from build123d import *

# Parameters (mm, degrees)
SKETCH1_W                                           = 160
SKETCH1_H                                           = 80
BOSS_EXTRUDE1_DEPTH                                 = 15
CBORE_FOR_M5_HEX_SOCKET_HEAD_CAP_SCREW1_D           = 5.5
CBORE_FOR_M5_HEX_SOCKET_HEAD_CAP_SCREW1_CBORE_D     = 10
CBORE_FOR_M5_HEX_SOCKET_HEAD_CAP_SCREW1_CBORE_DEPTH = 5.4
M6_TAPPED_HOLE1_D                                   = 5
SKETCH15_W                                          = 40
SKETCH15_H                                          = 80
SKETCH15_W_2                                        = 50
CUT_EXTRUDE1_DEPTH                                  = 2


with BuildPart() as part:
    # Sketch1 → Boss-Extrude1 (new body)
    with BuildSketch(Plane.XY):
        Rectangle(SKETCH1_W, SKETCH1_H)
    extrude(amount=BOSS_EXTRUDE1_DEPTH)

    # CBORE for M5 Hex Socket Head Cap Screw1 (through all)
    with Locations(Plane(origin=(74, 31, 0), x_dir=(-1, 0, 0), z_dir=(0, 0, -1))):
        with Locations((0, 0), (28, 0), (0, -21), (28, -21), (0, -41), (0, -62), (28, -41), (28, -62), (56, -41), (56, -21), (92, -21), (92, -41), (120, 0), (120, -21), (148, 0), (148, -21), (120, -41), (120, -62), (148, -41), (148, -62)):
            CounterBoreHole(CBORE_FOR_M5_HEX_SOCKET_HEAD_CAP_SCREW1_D / 2, CBORE_FOR_M5_HEX_SOCKET_HEAD_CAP_SCREW1_CBORE_D / 2, CBORE_FOR_M5_HEX_SOCKET_HEAD_CAP_SCREW1_CBORE_DEPTH)

    # M6 Tapped Hole1 (through all)
    with Locations(Plane(origin=(-60, -40, 7.5), x_dir=(0, 0, -1), z_dir=(0, -1, 0))):
        with Locations((0, 0), (0, 120)):
            Hole(M6_TAPPED_HOLE1_D / 2)

    # Sketch15 → Cut-Extrude1 (cut)
    with BuildSketch(Plane.XY.offset(15)):
        with Locations((-60, 0)):
            Rectangle(SKETCH15_W, SKETCH15_H)
        with Locations((60, 0)):
            Rectangle(SKETCH15_W, SKETCH15_H)
        Rectangle(SKETCH15_W_2, SKETCH15_H)
    extrude(amount=-CUT_EXTRUDE1_DEPTH, mode=Mode.SUBTRACT)


solid = part.part
The listing builds one solid part. Answer for the finished solid, in the listing's coordinates (mm). A direction names the side the tool comes from. Round coordinates to 2 decimals unless told otherwise and drop trailing zeros. Loops run counter-clockwise (first coordinate to the right, second up) from the corner with the lowest first, then second, coordinate; pieces in that order, holes last. Notation, with made-up numbers: M 74,37.5 L 113,37.5 A11 cw 113,52.5 Z; hole C 21,1.25 d5. An arc over 180 degrees is marked long. Return JSON: item names as keys, results as strings.
Q1. Find section A-A, the plane x = 60. Determine the outline of the cut face in (y, z), plus the area to 3 significant figures.
Results list:
{"outline": "M -40,0 L 40,0 L 40,5 L -40,5 Z; M -40,10 L 40,10 L 40,13 L -40,13 Z", "area": "640 mm2"}
Q2. Find the intervals of material crossed by line 1 along X through (y, z) = (31.5, 1.75); line 2 along Y through (x, z) = (-17.5, 2.25); line 3 along X through (y, z) = (1.5, 7.5), in increasing order. Write a range as from..to.
Results list:
{"line 1": "x = -80..-78.97, -69.03..-50.97, -41.03..41.03, 50.97..69.03, 78.97..80", "line 2": "y = -40..-14.97, -5.03..5.03, 14.97..40", "line 3": "x = -80..-62.5, -57.5..57.5, 62.5..80"}
Q3. The mould has two halves that part along Y. Classify faces 4 (the face through (-42, 13, 3)), 5 (the face through (-1, 40, 7)), 6 (the face through (32, 1, 15)): released by +Y, released by -Y, zero draft, split by the parting line, or undercut.
Results list:
{"face 4": "undercut", "face 5": "released by +Y", "face 6": "zero draft"}
Q4. Each of these flat-tipped pins is pushed along its axis until it touches: pin 1 Ø12 at (x, y) = (1.5, -16.5) entering from +Z; pin 2 Ø6 at (x, y) = (46, -31) entering from -Z; pin 3 Ø3 at (x, y) = (58, 6.5) entering from -Z; pin 4 Ø0.6 at (y, z) = (15.5, 14) entering from -X. Where does it stop, or does it pass through?
Results list:
{"pin 1": "stops at z = 13", "pin 2": "stops at z = 5.4", "pin 3": "stops at z = 0", "pin 4": "stops at x = -40"}
Q5. Find section D-D, the plane y = 0. Determine the outline of the cut face in (x, z), plus the area to 3 significant figures.
Results list:
{"outline": "M -80,0 L 80,0 L 80,13 L 40,13 L 40,15 L 25,15 L 25,13 L -25,13 L -25,15 L -40,15 L -40,13 L -80,13 Z; hole C -60,7.5 d5; hole C 60,7.5 d5", "area": "2,100 mm2"}
Q6. Find section C-C, the plane z = 1.5. State how many separate pieces and enclosed holes the cut face has, plus the area to 3 significant figures.
Results list:
{"separate pieces": "1", "enclosed holes": "20", "area": "11,200 mm2"}
Q7. Find section B-B, the plane x = 18. Determine the outline of the cut face in (y, z).
Results list:
{"outline": "M -40,0 L -15,0 L -15,5.4 L -12.75,5.4 L -12.75,13 L -40,13 Z; M -7.25,5.4 L -5,5.4 L -5,0 L 5,0 L 5,5.4 L 7.25,5.4 L 7.25,13 L -7.25,13 Z; M 12.75,5.4 L 15,5.4 L 15,0 L 40,0 L 40,13 L 12.75,13 Z"}
Q8. Which of the six approach directions +Z, -Z, +X, -X, +Y, -Y give full straight-line access (tool end or side, diameter ignored) to faces 1 (the face through (-60, 1, 13)), 2 (the face through (50, -34, 3)), 3 (the face through (43.253, -30.879, 9.253))?
Results list:
{"face 1": "+Z, -X, +Y, -Y", "face 2": "-Z", "face 3": "+Z, -Z"}
